Could you check a few things on this model? Use its own coordinates, in mm. A direction names the side the tool comes from. Give positions to 0.01 mm unless a question says otherwise; leave off trailing zeros. Loops run counter-clockwise (first coordinate to the right, second up) from the corner with the lowest first, then second, coordinate; pieces in that order, holes last. Notation, with made-up numbers: M 34.25,80 L 81.25,80 A16 cw 81.25,107 Z; hole C -23.5,-10.5 d2. An arc over 180 degrees is marked long. Answer in a Markdown table with one row per item. Add a question column.
```python
from build123d import *

# Parameters (mm, degrees)
F0_R     = 4
F1_DEPTH = 3
F2_R     = 6
F3_DEPTH = 10
F4_R     = 2.5
F5_DEPTH = 2
F6_R     = 1.99999
F7_R     = 2.5
F8_DEPTH = 8


# Not quite as in the source:
# - a fillet or chamfer is up to 0.001 mm smaller than in the source, because OpenCascade refuses the exact size


with BuildPart() as f1:
    # F0 (on Top) → F1 (new body)
    with BuildSketch(Plane.XY):
        Circle(F0_R)
    extrude(amount=F1_DEPTH)

    # F2 (on face) → F3 (join)
    with BuildSketch(Plane.XY.offset(3)):
        Circle(F2_R)
    extrude(amount=F3_DEPTH)

    # F4 (on face) → F5 (join)
    with BuildSketch(Plane.XY.offset(13)):
        Circle(F4_R)
    extrude(amount=F5_DEPTH)

    # F6 (radius 2 in the source; OpenCascade refuses exactly that, so slightly less here)
    f6_edges = [f1.edges().sort_by_distance(p)[0] for p in [
        (-6, 0, 13),
        (-6, 0, 3),
    ]]
    fillet(f6_edges, radius=F6_R)

    # F7 (on face) → F8 (cut)
    with BuildSketch(Plane(origin=(0, 0, 0), x_dir=(1, 0, 0), z_dir=(0, 0, -1))):
        Circle(F7_R)
    extrude(amount=-F8_DEPTH, mode=Mode.SUBTRACT)


solid = f1.part
```
Item 1: For P1, Ø1, axis at x = 2, z = 12.5, coming from the +Y side; P2, Ø2, axis at y = -2, z = 10, coming from the +X side; P3, Ø6, axis at y = -4.5, z = 11, coming from the +X side, each with a flat end and sliding along its axis, tell me the tip position at first contact or that it passes through.
Item 2: I need wall thicknesses on L1, parallel to Y at x = 0, z = 2.5; L2, parallel to Z at x = 2.5, y = 2.5; L3, parallel to Y at x = 0, z = 5.5. Which ranges of each line are inside material? Lowest first, please.
Item 3: If we mould it in two halves opening along Y, with no side actions, what happens to faces 4 (the face through (2, 2, 0)), 5 (the face through (-0.54, 2.44, 3.94)), 6 (the face through (-0.54, -2.44, 13.99)), 7 (the face through (0, 0, 8))? For each: +Y half, -Y half, draft (parallel to the pull), parting line (faces both ways), or undercut.
Item 4: Suppose I cut it at D-D (z = 5.5). List the corners of the cut face in (x, y) for me, then the cut area to 3 significant figures.
Item 5: Suppose I cut it at C-C (z = 13.5). List the corners of the cut face in (x, y) for me.
Item 6: For faces 1 (the face through (-0.867, -3.905, 1.479)), 2 (the face through (-6, 0, 8)), 3 (the face through (-2, -2, 13)), which set-ups out of +Z, -Z, +X, -X, +Y, -Y let a thin tool reach every point of the face, with its end or its side?
Values found:
| question | item | result |
|---|---|---|
| 1 | P1 | y = 5.42 |
| 1 | P2 | x = 5.92 |
| 1 | P3 | x = 5.81 |
| 2 | L1 | -4 to -2.5, 2.5 to 4 |
| 2 | L2 | 0 to 13 |
| 2 | L3 | -6 to -2.5, 2.5 to 6 |
| 3 | face 4 | draft |
| 3 | face 5 | undercut |
| 3 | face 6 | parting line |
| 3 | face 7 | undercut |
| 4 | outline | C 0,0 d12; hole C 0,0 d5 |
| 4 | area | 93.5 mm² |
| 5 | outline | C 0,0 d5 |
| 6 | face 1 | -Z |
| 6 | face 2 | +Z, -Z |
| 6 | face 3 | +Z |
